The model under review builds one solid part; all positions refer to its coordinate system, in mm. Give positions to 0.01 mm unless a question says otherwise; leave off trailing zeros. Order: outer loops, then holes, each group sorted by start corner. A loop starts at its lowest first (then second) coordinate and runs counter-clockwise, first axis right, second up. Notation, with made-up numbers: (-31.75, 82) - (10.25, 82) arc R23 ccw to (10.25, 95) - close; hole circle Ø3 at (-10.5, 40). An arc over 180 degrees is marked (long way). Put each result on its own line as item: value.
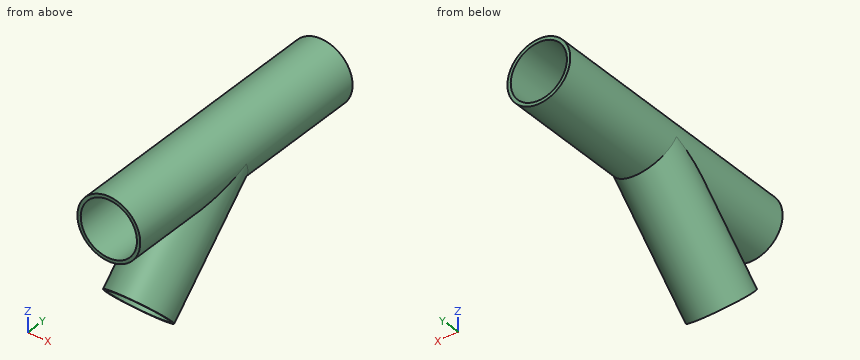
```python
from build123d import *

# Parameters (mm, degrees)
SALIENTE_EXTRUIR1_DEPTH      = 125
SALIENTE_EXTRUIR1_DEPTH_BACK = 125
CROQUIS1_R                   = 28.4
CROQUIS1_R_2                 = 25.4
CROQUIS4_R                   = 28.4
CROQUIS4_R_2                 = 25.4
SALIENTE_EXTRUIR3_DEPTH      = 125


with BuildPart() as part:
    # Croquis1 → Saliente-Extruir1 (new, two sides: drawn at the far end of the back side and taken through both)
    with BuildSketch(Plane(origin=(0, 0, 0), x_dir=(1, 0, 0), z_dir=(0, 1, 0)).offset(-SALIENTE_EXTRUIR1_DEPTH_BACK)):
        with Locations(Location((0, 0, 0), (0, 0, 270))):
            Circle(CROQUIS1_R)
        with Locations(Location((0, 0, 0), (0, 0, 270))):
            Circle(CROQUIS1_R_2, mode=Mode.SUBTRACT)
    extrude(amount=SALIENTE_EXTRUIR1_DEPTH + SALIENTE_EXTRUIR1_DEPTH_BACK)

    # Croquis4 → Saliente-Extruir3 (add)
    with BuildSketch(Plane(origin=(0, 0, 0), x_dir=(0, 0.6946583704589961, -0.7193398003386523), z_dir=(0, -0.7193398003386523, -0.6946583704589961))):
        with Locations(Location((0, 0, 0), (0, 0, 90))):
            Circle(CROQUIS4_R)
        with Locations(Location((0, 0, 0), (0, 0, 180))):
            Circle(CROQUIS4_R_2, mode=Mode.SUBTRACT)
    extrude(amount=SALIENTE_EXTRUIR3_DEPTH)


solid = part.part
```
(1) Take a section at A-A, the plane x = 4. Write out the cut boundary in (y, z).
The answers:
outline: (-125, -28.12) - (-69.59, -28.12) - (-109.45, -66.61) - (-107.34, -68.79) - (-65.22, -28.12) - (6.99, -28.12) - (-72.49, -104.88) - (-70.39, -107.06) - (11.36, -28.12) - (125, -28.12) - (125, -25.08) - (14.5, -25.08) - (19.53, -20.23) - (17.42, -18.04) - (10.13, -25.08) - (-62.08, -25.08) - (-17.42, 18.04) - (-19.53, 20.23) - (-66.45, -25.08) - (-125, -25.08) - close; (-125, 25.08) - (125, 25.08) - (125, 28.12) - (-125, 28.12) - close
(2) Take a section at C-C, the plane x = -9. Write out the cut boundary in (y, z).
The answers:
outline: (-125, -26.94) - (-66.67, -26.94) - (-108.63, -67.46) - (-106.42, -69.75) - (-62.09, -26.94) - (6.3, -26.94) - (-73.42, -103.92) - (-71.21, -106.21) - (10.88, -26.94) - (125, -26.94) - (125, -23.75) - (14.18, -23.75) - (18.71, -19.38) - (16.5, -17.09) - (9.6, -23.75) - (-58.79, -23.75) - (-16.5, 17.09) - (-18.71, 19.38) - (-63.37, -23.75) - (-125, -23.75) - close; (-125, 23.75) - (125, 23.75) - (125, 26.94) - (-125, 26.94) - close
(3) Take a section at D-D, the plane y = 2.5. Count the separate pieces of the cut face and the enclosed holes in it, then the cut area to 3 significant figures.
The answers:
separate pieces: 1
enclosed holes: 2
area: 747 mm^2
(4) Take a section at B-B, the plane y = 85. Write out the cut boundary in (x, z), then the cut area to 3 significant figures.
The answers:
outline: circle Ø56.8 at (0, 0); hole circle Ø50.8 at (0, 0)
area: 507 mm^2
(5) Clearance check with flat-ended pins moving along their axes: pin 1 Ø1 at (x, y) = (-19, 81.5) entering from -Z; pin 2 Ø1 at (x, z) = (-18, -23) entering from +Y; pin 3 Ø10 at (y, z) = (-66, -38.5) entering from +X. State where each tip first meets the part, or that it passes through.
The answers:
pin 1: z = -21.55
pin 2: y = 8.58
pin 3: x = 25.17
(6) Wall thickness on L1, parallel to X at y = 56, z = 0; L2, parallel to Z at x = -10, y = 15.5; L3, parallel to Z at x = -11, y = 80: over which ranges is each line inside the solid? List them lowest first.
The answers:
L1: -28.4 to -25.4, 25.4 to 28.4
L2: -26.58 to -23.35, -21.98 to -17.49, 23.35 to 26.58
L3: -26.18 to -22.89, 22.89 to 26.18
